The figure shows three views and two pictorial views of one solid part (mm, origin at its lowest corner). Answer the questions. A direction names the side the tool comes from. Round coordinates to 2 decimals unless told otherwise and drop trailing zeros. Order: outer loops, then holes, each group sorted by start corner. A loop starts at its lowest first (then second) coordinate and runs counter-clockwise, first axis right, second up. Notation, with made-up numbers: (-14, 47.5) - (22, 47.5) arc R22 ccw to (22, 85.5) - close; hole circle Ø11 at (39, -30.5). An arc over 180 degrees is marked (long way). Write item = value, one per line.
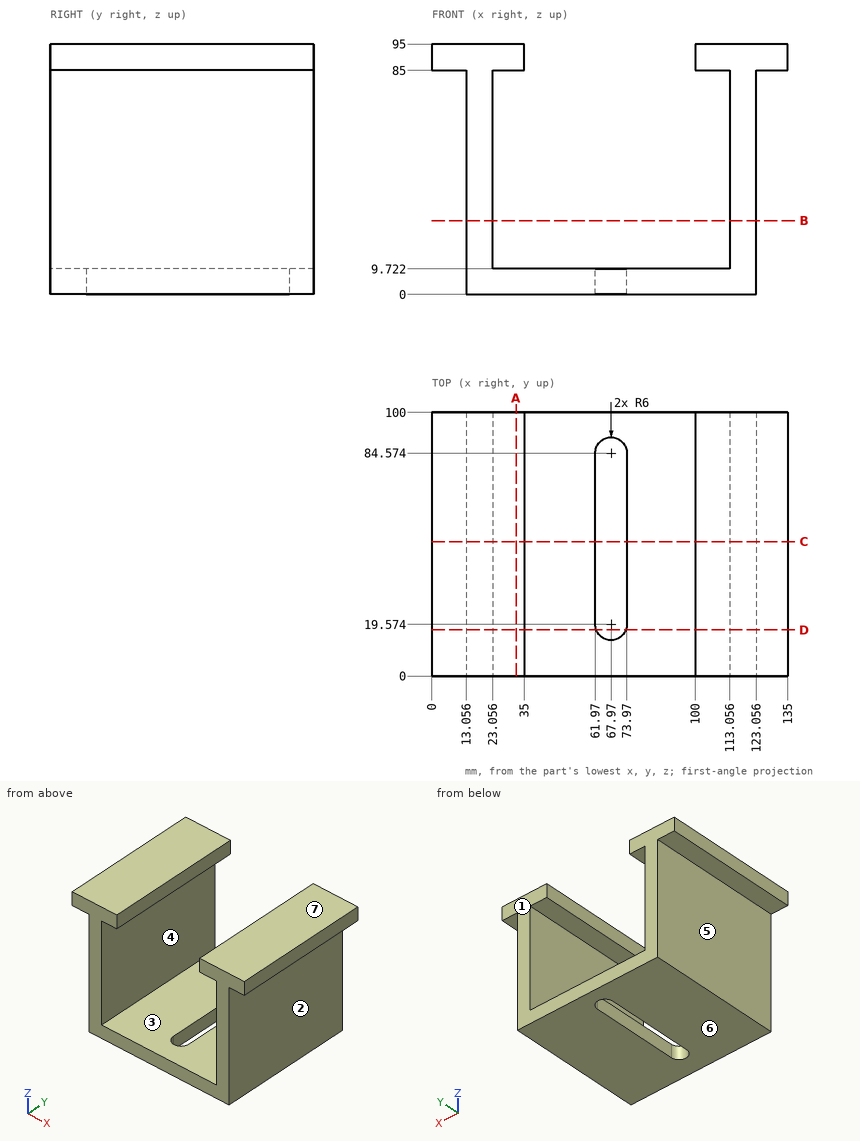
Q1. Section C-C on y = 51 is taken. Determine the outline of the cut face in (x, z) (1 decimal), then the cut area to 3 significant figures.
Model answer:
outline = (0, 85) - (13.1, 85) - (13.1, 0) - (62, 0) - (62, 9.7) - (23.1, 9.7) - (23.1, 85) - (35, 85) - (35, 95) - (0, 95) - close; (74, 0) - (123.1, 0) - (123.1, 85) - (135, 85) - (135, 95) - (100, 95) - (100, 85) - (113.1, 85) - (113.1, 9.7) - (74, 9.7) - close
area = 3,160 mm^2
Q2. Determine the mould class of the marked faces 4, 5, 6 and 7 for opening direction Z: released by +Z, released by -Z, zero draft, split by the parting line, or undercut.
Model answer:
face_4 = undercut
face_5 = zero draft
face_6 = released by -Z
face_7 = released by +Z
Q3. For the marked faces 1, 2 and 3, determine the directions among +Z, -Z, +X, -X, +Y, -Y from which every point of the face is accessible in a straight line to the end or side of a thin tool.
Model answer:
face_1 = +Z, -Z, +X, -X, +Y
face_2 = -Z, +X, +Y, -Y
face_3 = +Y, -Y
Q4. Find the intervals of material crossed by line 1 (X direction, y = 20.5, z = 32.5) (1 decimal); line 2 (Z direction, x = 104, y = 22.5); line 3 (X direction, y = 74.5, z = 9) (1 decimal), in increasing order. Write a range as from..to.
Model answer:
line_1 = 13.1..23.1, 113.1..123.1
line_2 = 0..9.72, 85..95
line_3 = 13.1..62, 74..123.1
Q5. Flat-ended cylindrical pins translate along their axes: P1, Ø9.5, axis at x = 126.5, y = 44, coming from the -Z side; P2, Ø4, axis at y = 66, z = 14, coming from the +X side; P3, Ø22.5, axis at y = 74, z = 62, coming from the -X side; P4, Ø1.5, axis at x = 56.5, y = 77, coming from the +Z side. Find the tip coordinate at first contact, or state that the pin passes through.
Model answer:
P1 = 0
P2 = 123.06
P3 = 13.06
P4 = 9.72
Q6. Section B-B on z = 28 is taken. Determine the outline of the cut face in (x, y) (1 decimal).
Model answer:
outline = (13.1, 0) - (23.1, 0) - (23.1, 100) - (13.1, 100) - close; (113.1, 0) - (123.1, 0) - (123.1, 100) - (113.1, 100) - close
Q7. Section A-A on x = 32 is taken. Determine the outline of the cut face in (y, z).
Model answer:
outline = (0, 0) - (100, 0) - (100, 9.72) - (0, 9.72) - close; (0, 85) - (100, 85) - (100, 95) - (0, 95) - close
Q8. Section D-D on y = 17.5 is taken. Determine the outline of the cut face in (x, z) (1 decimal).
Model answer:
outline = (0, 85) - (13.1, 85) - (13.1, 0) - (62.3, 0) - (62.3, 9.7) - (23.1, 9.7) - (23.1, 85) - (35, 85) - (35, 95) - (0, 95) - close; (73.6, 0) - (123.1, 0) - (123.1, 85) - (135, 85) - (135, 95) - (100, 95) - (100, 85) - (113.1, 85) - (113.1, 9.7) - (73.6, 9.7) - close
